Geometry: final body of the model. Coordinates: model frame, mm. Give positions to 0.01 mm unless a question says otherwise; leave off trailing zeros. Write each loop counter-clockwise with the first axis right and the second up, starting at its lowest first coordinate (ties: lowest second). Pieces come first, ordered by that corner, then holes.
Q1. Cut plane B-B on z = 478. Return the cut outline in (x, y).
Q2. Draft query along Y for faces 1 (the face through (4, 53.944, 466)), 2 (the face through (4, 47, 446.407)), 3 (the face through (3.944, 47.72, 481.903)). Return one class per face: pulls with the +Y half, pulls with the -Y half, needs draft (parallel to the pull), parting line crosses it, or undercut.
Q3. Pin query (flat end, axial travel): pin 1 (3 mm diameter, centred on y = 46, z = 475.5, fed in from +X). Return the tip coordinate at first contact, or that it passes through.
Q4. Line query: L1, parallel to Z at x = 4.5, y = 46.25; L2, parallel to Z at x = 2.25, y = 45.25; L3, parallel to Y at x = 7.5, z = 480.5. Output: solid intervals per line, ascending.
Q5. Cut plane D-D on y = 46.5. Return the cut outline in (x, z), plus the area to 3 significant figures.
Q6. Cut plane C-C on x = 5. Return the cut outline in (y, z).
Q7. Cut plane A-A on y = 49.25. Return the cut outline in (x, z), plus the area to 3 significant figures.
```python
from build123d import *

# Parameters (mm, degrees)
SKETCH1_W           = 38
SKETCH1_H           = 13
SKETCH1_R           = 4
BOSS_EXTRUDE1_DEPTH = 8


with BuildPart() as part:
    # Sketch1 → Boss-Extrude1 (new body)
    with BuildSketch(Plane(origin=(0, 0, 0), x_dir=(0, 0, -1), z_dir=(1, 0, 0))):
        with Locations((-465.406543956, 47.44372232)):
            Rectangle(SKETCH1_W, SKETCH1_H)
        with Locations((-477.906543956, 47.54372232)):
            Circle(SKETCH1_R, mode=Mode.SUBTRACT)
        with Locations((-452.906543956, 47.54372232)):
            Circle(SKETCH1_R, mode=Mode.SUBTRACT)
    extrude(amount=BOSS_EXTRUDE1_DEPTH)


solid = part.part
```
Data:
1. outline: (0, 40.94) - (8, 40.94) - (8, 43.54) - (0, 43.54) - close; (0, 51.54) - (8, 51.54) - (8, 53.94) - (0, 53.94) - close
2. face 1: pulls with the +Y half
2. face 2: needs draft
2. face 3: undercut
3. pin 1: stops at x = 8
4. L1: z = 446.41 to 449.12, 456.69 to 474.12, 481.69 to 484.41
4. L2: z = 446.41 to 449.63, 456.18 to 474.63, 481.18 to 484.41
4. L3: y = 40.94 to 44.5, 50.59 to 53.94
5. outline: (0, 446.41) - (8, 446.41) - (8, 449.05) - (0, 449.05) - close; (0, 456.77) - (8, 456.77) - (8, 474.05) - (0, 474.05) - close; (0, 481.77) - (8, 481.77) - (8, 484.41) - (0, 484.41) - close
5. area: 180 mm2
6. outline: (40.94, 446.41) - (53.94, 446.41) - (53.94, 484.41) - (40.94, 484.41) - close; hole circle Ø8 at (47.54, 452.91); hole circle Ø8 at (47.54, 477.91)
7. outline: (0, 446.41) - (8, 446.41) - (8, 449.29) - (0, 449.29) - close; (0, 456.52) - (8, 456.52) - (8, 474.29) - (0, 474.29) - close; (0, 481.52) - (8, 481.52) - (8, 484.41) - (0, 484.41) - close
7. area: 188 mm2
